The figure shows three views and two pictorial views of one solid part (mm, origin at its lowest corner). Answer the questions. Give positions to 0.01 mm unless a question says otherwise; leave off trailing zeros. Order: outer loops, then holes, each group sorted by start corner. A loop starts at its lowest first (then second) coordinate and runs counter-clockwise, first axis right, second up. Notation, with made-up numbers: (8.5, -23) - (19.5, -23) arc R21 ccw to (19.5, -1) - close; hole circle Ø5 at (-31.75, 49.5). An arc over 180 degrees is marked (long way). Use a Markdown table: item, result. Add a question column.
1. Consider L1, parallel to X at y = 13, z = 30 (3 decimals); L2, parallel to Y at x = 13.75, z = 19; L3, parallel to Z at x = 18.75, y = 18. Determine where each line is inside the solid, lowest interval first.
2. For a pull along X with two mould halves and no side action, classify the marked faces 1, 2 and 3 as released by +X, released by -X, zero draft, split by the parting line, or undercut.
3. Flat-ended cylindrical pins translate along their axes: P1, Ø1, axis at x = 7.5, z = 16.5, coming from the -Y side; P2, Ø5, axis at x = 6.5, z = 21, coming from the +Y side; P3, Ø10, axis at x = 22, y = 21.5, coming from the +Z side. Find the tip coordinate at first contact, or state that the pin passes through.
4. A cutting plane is placed at A-A on x = 13.5. Determine the outline of the cut face in (y, z) (3 decimals).
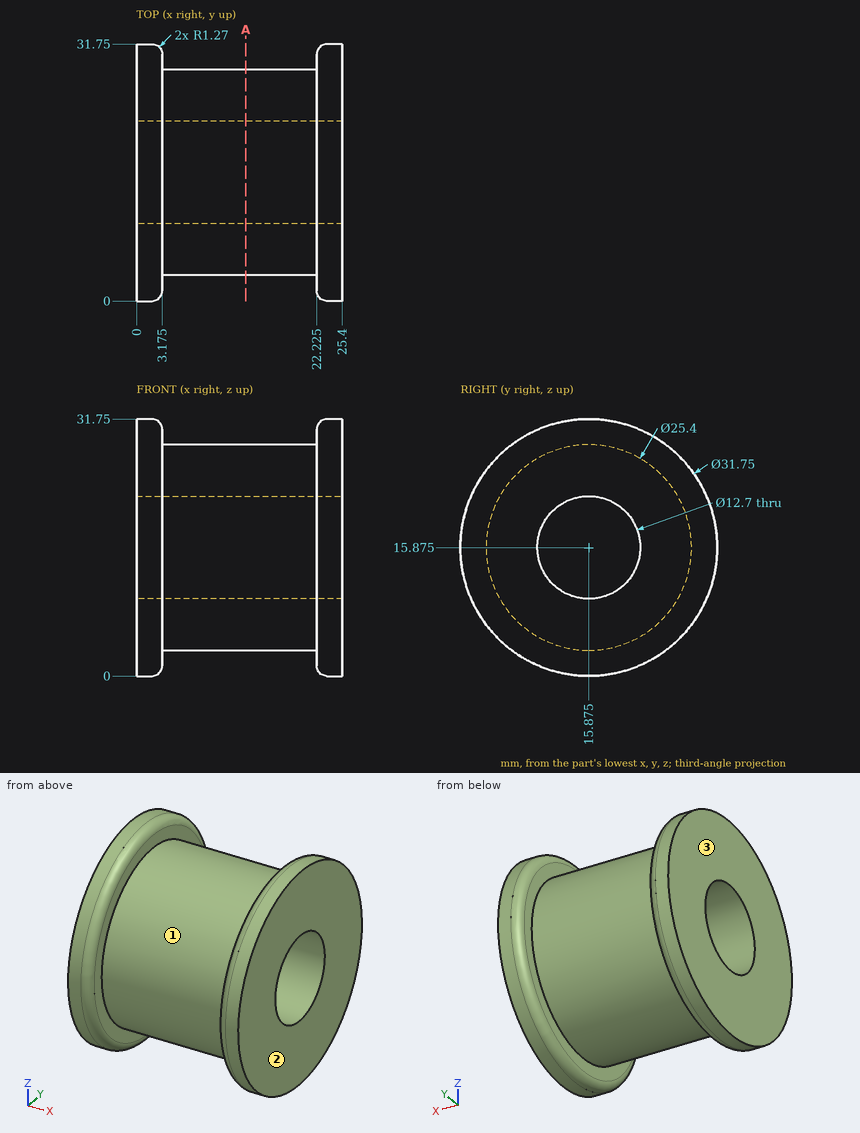
Output values:
| question | item | result |
|---|---|---|
| 1 | L1 | 0 to 3.175, 22.225 to 25.4 |
| 1 | L2 | 3.57 to 10.35, 21.4 to 28.18 |
| 1 | L3 | 3.35 to 9.89, 21.86 to 28.4 |
| 2 | face 1 | undercut |
| 2 | face 2 | released by +X |
| 2 | face 3 | released by -X |
| 3 | P1 | y = 3.18 |
| 3 | P2 | y = 28.3 |
| 3 | P3 | z = 31.73 |
| 4 | outline | circle Ø25.4 at (15.875, 15.875); hole circle Ø12.7 at (15.875, 15.875) |
